Source: CAD feature listing. Evaluate the final solid. Frame: model axes, mm. Face numbers are marked on the shaded views. Give positions to 0.01 mm unless a question says otherwise; leave off trailing zeros. Order: outer loops, then holes, each group sorted by start corner. A loop starts at its lowest first (then second) coordinate and runs counter-clockwise, first axis right, second up. Notation, with made-up numbers: (67.25, 46.25) -> (84.25, 46.25) arc R23 ccw to (84.25, 58.25) -> close; hole circle Ø2 at (-4, 34). An arc over 180 degrees is marked (long way). Use CSV: the item, a comma, the result in double quotes.
```python
from build123d import *

# Parameters (mm, degrees)
BOSS_EXTRUDE1_DEPTH = 3
SKETCH2_R           = 2.75
CUT_EXTRUDE1_DEPTH  = 4
SKETCH3_R           = 5.75
SKETCH3_R_2         = 2.75
BOSS_EXTRUDE2_DEPTH = 4.5
SKETCH4_R           = 2.25
CUT_EXTRUDE2_DEPTH  = 4


with BuildPart() as part:
    # Sketch1 → Boss-Extrude1 (new body)
    with BuildSketch(Plane(origin=(0, 0, 0), x_dir=(1, 0, 0), z_dir=(0, 1, 0))):
        with BuildLine():
            Line((-55, 10), (6.534997659, 10))
            ThreePointArc((6.534997659, 10), (9.382971848, 10.890371912), (11.216643547, 13.244382792))
            Line((11.216643547, 13.244382792), (23.783356453, 46.755617208))
            ThreePointArc((23.783356453, 46.755617208), (25.617028152, 49.109628088), (28.465002341, 50))
            Line((28.465002341, 50), (41.279846746, 50))
            ThreePointArc((41.279846746, 50), (44.264499394, 49.011464641), (46.068978172, 46.436739428))
            Line((46.068978172, 46.436739428), (59.568978172, 1.436739428))
            ThreePointArc((59.568978172, 1.436739428), (59.779846746, 0), (59.568978172, -1.436739428))
            Line((59.568978172, -1.436739428), (46.068978172, -46.436739428))
            ThreePointArc((46.068978172, -46.436739428), (44.264499394, -49.011464641), (41.279846746, -50))
            Line((41.279846746, -50), (28.465002341, -50))
            ThreePointArc((28.465002341, -50), (25.617028152, -49.109628088), (23.783356453, -46.755617208))
            Line((23.783356453, -46.755617208), (11.216643547, -13.244382792))
            ThreePointArc((11.216643547, -13.244382792), (9.382971848, -10.890371912), (6.534997659, -10))
            Line((6.534997659, -10), (-55, -10))
            ThreePointArc((-55, -10), (-58.535533906, -8.535533906), (-60, -5))
            Line((-60, -5), (-60, 5))
            ThreePointArc((-60, 5), (-58.535533906, 8.535533906), (-55, 10))
        make_face()
    extrude(amount=BOSS_EXTRUDE1_DEPTH)

    # Sketch2 → Cut-Extrude1 (cut, through all)
    with BuildSketch(Plane(origin=(0, 3, 0), x_dir=(1, 0, 0), z_dir=(0, 1, 0))):
        with Locations((-27, 0)):
            Circle(SKETCH2_R)
        with Locations((35, 40)):
            Circle(SKETCH2_R)
        with Locations((35, -40)):
            Circle(SKETCH2_R)
    extrude(amount=-CUT_EXTRUDE1_DEPTH, mode=Mode.SUBTRACT)

    # Sketch3 → Boss-Extrude2 (add)
    with BuildSketch(Plane(origin=(0, 3, 0), x_dir=(1, 0, 0), z_dir=(0, 1, 0))):
        with Locations((-27, 0)):
            Circle(SKETCH3_R)
        with Locations((-27, 0)):
            Circle(SKETCH3_R_2, mode=Mode.SUBTRACT)
        with Locations((35, 40)):
            Circle(SKETCH3_R)
        with Locations((35, 40)):
            Circle(SKETCH3_R_2, mode=Mode.SUBTRACT)
        with Locations((35, -40)):
            Circle(SKETCH3_R)
        with Locations((35, -40)):
            Circle(SKETCH3_R_2, mode=Mode.SUBTRACT)
    extrude(amount=BOSS_EXTRUDE2_DEPTH)

    # Sketch4 → Cut-Extrude2 (cut, through all)
    with BuildSketch(Plane(origin=(0, 3, 0), x_dir=(1, 0, 0), z_dir=(0, 1, 0))):
        with Locations((-55, 0)):
            Circle(SKETCH4_R)
        with Locations((45, 0)):
            Circle(SKETCH4_R)
        with Locations((-7, 0)):
            Circle(SKETCH4_R)
    extrude(amount=-CUT_EXTRUDE2_DEPTH, mode=Mode.SUBTRACT)


solid = part.part
```
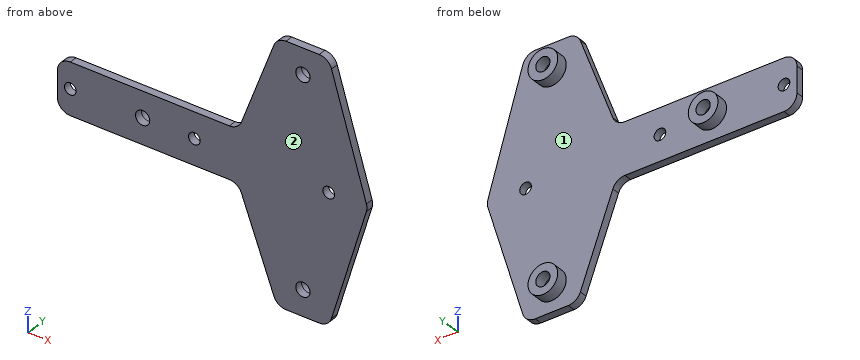
1. Section query B-B on y = 5. Return loops of the section in (x, z).
Answer below:
outline,"circle Ø11.5 at (-27, 0); circle Ø11.5 at (35, -40); circle Ø11.5 at (35, 40); hole circle Ø5.5 at (-27, 0); hole circle Ø5.5 at (35, -40); hole circle Ø5.5 at (35, 40)"
2. Section query D-D on x = -7. Return loops of the section in (y, z).
Answer below:
outline,"(0, -10) -> (3, -10) -> (3, -2.25) -> (0, -2.25) -> close; (0, 2.25) -> (3, 2.25) -> (3, 10) -> (0, 10) -> close"
3. Ray query, line 1 along Z through (x, y) = (35, 3.5); line 2 along Z through (x, y) = (35, 2.25); line 3 along Z through (x, y) = (-27, 1.75). Return the intervals inside material, ascending.
Answer below:
line 1,"z = -45.75 to -42.75, -37.25 to -34.25, 34.25 to 37.25, 42.75 to 45.75"
line 2,"z = -50 to -42.75, -37.25 to 37.25, 42.75 to 50"
line 3,"z = -10 to -2.75, 2.75 to 10"
4. Section query A-A on x = 35. Return loops of the section in (y, z), plus the area to 3 significant figures.
Answer below:
outline,"(0, -50) -> (3, -50) -> (3, -45.75) -> (7.5, -45.75) -> (7.5, -42.75) -> (0, -42.75) -> close; (0, -37.25) -> (7.5, -37.25) -> (7.5, -34.25) -> (3, -34.25) -> (3, 34.25) -> (7.5, 34.25) -> (7.5, 37.25) -> (0, 37.25) -> close; (0, 42.75) -> (7.5, 42.75) -> (7.5, 45.75) -> (3, 45.75) -> (3, 50) -> (0, 50) -> close"
area,"321 mm²"
5. Mould query, pull axis Z, two halves, no side actions, for the marked faces 1 and 2. Classes: released by +Z, released by -Z, zero draft, split by the parting line, or undercut.
Answer below:
face 1,"undercut"
face 2,"zero draft"
6. Section query C-C on z = 40. Return loops of the section in (x, y), plus the area to 4 significant figures.
Answer below:
outline,"(21.25, 0) -> (32.25, 0) -> (32.25, 7.5) -> (29.25, 7.5) -> (29.25, 3) -> (21.25, 3) -> close; (37.75, 0) -> (48, 0) -> (48, 3) -> (40.75, 3) -> (40.75, 7.5) -> (37.75, 7.5) -> close"
area,"90.75 mm²"
7. Pin query (flat end, axial travel): P1, Ø4.5, axis at x = -27, z = 0, coming from the -Y side; P2, Ø0.9, axis at x = -23, y = 1, coming from the +Z side; P3, Ø3, axis at x = -34, y = 1, coming from the -Z side; P4, Ø6, axis at x = 43, z = -33, coming from the +Y side. Return the tip coordinate at first contact, or that it passes through.
Answer below:
P1,"passes through"
P2,"stops at z = 10"
P3,"stops at z = -10"
P4,"stops at y = 3"
